from build123d import *

# Parameters (mm, degrees)
BOSS_EXTRUDE1_DEPTH = 1.2
BOSS_EXTRUDE3_DEPTH = 2


# Read off the part's stored shape, not the designer's step: Boss-Extrude3
with BuildPart() as part:
    # Sketch1 → Boss-Extrude1 (new body)
    with BuildSketch(Plane.XY):
        Polygon((0, 0), (33, 0), (33, -1.2), (33, -30), (0, -30), (0, -1.2), align=None)
    extrude(amount=BOSS_EXTRUDE1_DEPTH)

    # Boss-Extrude3 outline → Boss-Extrude3 (add)
    with BuildSketch(Plane(origin=(33, 0, 0), x_dir=(0, 0, -1), z_dir=(1, 0, 0))):
        with BuildLine():
            ThreePointArc((0, -0.270849738), (-0.6, 0), (-1.2, -0.270849738))
            Line((-1.2, -0.270849738), (-1.2, -1.329150262))
            ThreePointArc((-1.2, -1.329150262), (-0.6, -1.6), (0, -1.329150262))
            Line((0, -1.329150262), (0, -0.270849738))
        make_face()
    boss_extrude3 = extrude(amount=BOSS_EXTRUDE3_DEPTH)

    # Mirror1: Boss-Extrude3 across plane
    add(boss_extrude3.mirror(Plane.ZY.offset(-16.5)))


solid = part.part
Here's how the part is built. I have some questions about the finished solid (model axes, mm). A direction names the side the tool comes from. Round coordinates to 2 decimals unless told otherwise and drop trailing zeros. Write each loop counter-clockwise with the first axis right and the second up, starting at its lowest first coordinate (ties: lowest second). Pieces come first, ordered by that corner, then holes.
1. For faces 1 (the cylindrical face through (-1, -1.6, 0.6)), 2 (the flat face through (33, -16, 1)), 3 (the flat face through (0, -15, 1)), 4 (the cylindrical face through (34, -1.6, 0.6)), which set-ups out of +Z, -Z, +X, -X, +Y, -Y let a thin tool reach every point of the face, with its end or its side?
2. Suppose I cut it at B-B (y = -10.25). List the corners of the cut face in (x, z) for me, and give its area (3 significant figures).
3. I need wall thicknesses on L1, parallel to X at y = -11.5, z = 1. Which ranges of the line are inside material? Lowest first, please.
Answer sheet:
1. face 1: -X, -Y
1. face 2: +Z, -Z, +X, -Y
1. face 3: +Z, -Z, -X, -Y
1. face 4: +X, -Y
2. outline: (0, 0) - (33, 0) - (33, 1.2) - (0, 1.2) - close
2. area: 39.6 mm2
3. L1: x = 0 to 33
